Here's the drawing with two shaded views (mm, measured from the low corner). I have some questions. A direction names the side the tool comes from. Give positions to 0.01 mm unless a question says otherwise; leave off trailing zeros. Loops run counter-clockwise (first coordinate to the right, second up) from the corner with the lowest first, then second, coordinate; pieces in that order, holes last. Notation, with made-up numbers: M 86.25,-14 L 93.25,-14 A17 cw 93.25,12 Z; hole C -26,66.5 d4. An arc over 180 degrees is marked long. Use a Markdown table: item, result. Add a question column.
1) Which directions (+Z, -Z, +X, -X, +Y, -Y) give clear straight access to the entire face, cutting with the end or side of a thin tool? Please do the marked faces 1, 2, 3 and 4.
2) Will these pins go through, and if not, where does the flat tip stop? pin 1 Ø5 at (x, z) = (10, 16) entering from +Y; pin 2 Ø13 at (y, z) = (25.5, 8) entering from +X; pin 3 Ø3 at (x, z) = (8.78, 19.72) entering from +Y (1 decimal).
3) Suppose I cut it at C-C on x = 2.25. List the corners of the cut face in (y, z) for me.
4) Suppose I cut it at D-D on y = 10. List the corners of the cut face in (x, z) for me, and give its area (3 significant figures).
5) We'd pull the mould along Z, two halves only. Please class the marked faces 5, 6 and 7: +Z half, -Z half, draft (parallel to the pull), parting line (faces both ways), or undercut.
6) Suppose I cut it at A-A on z = 6. List the corners of the cut face in (x, y) for me, and give its area (3 significant figures).
7) If I drill on line 1 along Y through (x, z) = (5.75, 8.75); line 2 along Z through (x, y) = (10.5, 18); line 3 along Y through (x, z) = (9.5, 6.5), over which ranges is the centre line in solid material (lowest first)? Write a range as [from, to].
8) Suppose I cut it at B-B on y = 27.25. List the corners of the cut face in (x, z) for me.
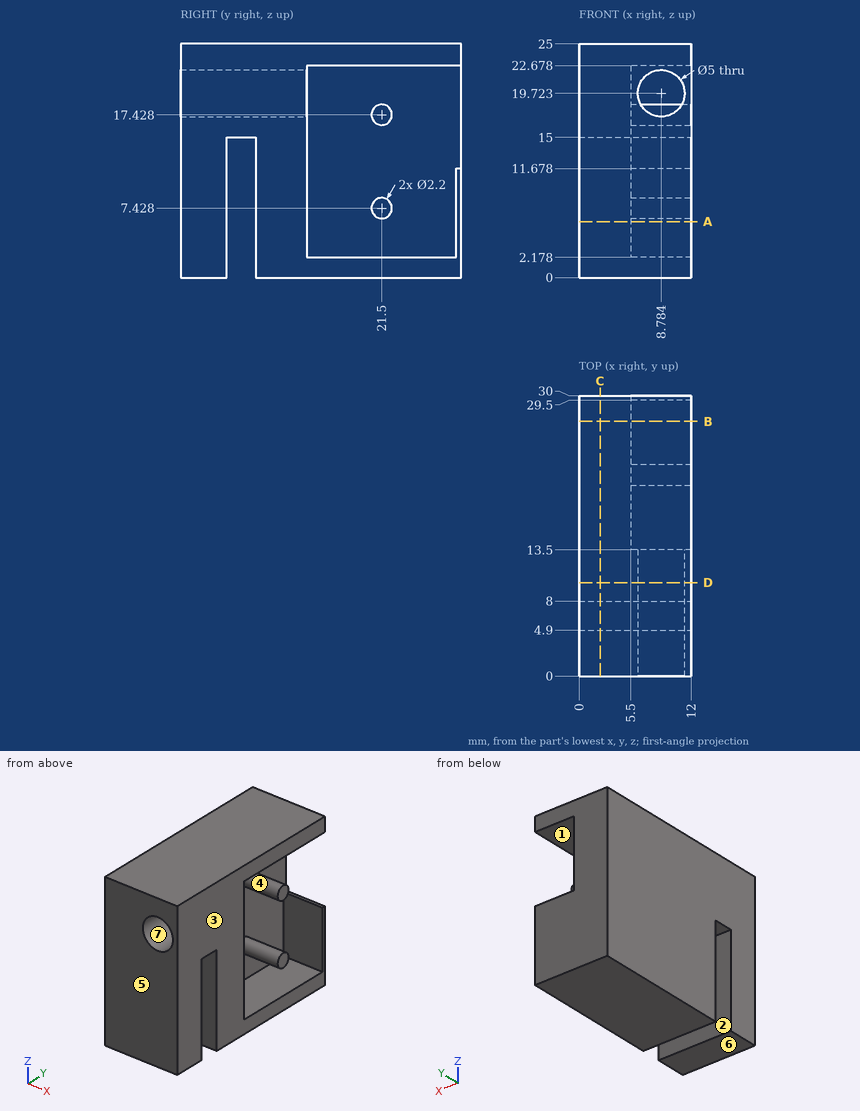
Answer block:
| question | item | result |
|---|---|---|
| 1 | face 1 | +X, +Y |
| 1 | face 2 | -Z, +X, -X |
| 1 | face 3 | +Z, -Z, +X, +Y, -Y |
| 1 | face 4 | +X |
| 2 | pin 1 | stops at y = 22.6 |
| 2 | pin 2 | stops at x = 12 |
| 2 | pin 3 | stops at y = 22.3 |
| 3 | outline | M 0,0 L 4.9,0 L 4.9,15 L 8,15 L 8,0 L 30,0 L 30,25 L 0,25 Z |
| 4 | outline | M 0,0 L 12,0 L 12,25 L 0,25 Z; hole C 8.78,19.72 d5 |
| 4 | area | 280 mm^2 |
| 5 | face 5 | draft |
| 5 | face 6 | -Z half |
| 5 | face 7 | undercut |
| 6 | outline | M 0,0 L 12,0 L 12,4.9 L 0,4.9 Z; M 0,8 L 12,8 L 12,13.5 L 5.5,13.5 L 5.5,29.5 L 12,29.5 L 12,30 L 0,30 Z |
| 6 | area | 219 mm^2 |
| 7 | line 1 | y = [0, 4.9], [8, 13.5], [29.5, 30] |
| 7 | line 2 | z = [0, 2.18], [22.68, 25] |
| 7 | line 3 | y = [0, 4.9], [8, 13.5], [20.91, 22.09], [29.5, 30] |
| 8 | outline | M 0,0 L 12,0 L 12,2.18 L 5.5,2.18 L 5.5,22.68 L 12,22.68 L 12,25 L 0,25 Z |
